For this review, take the finished solid that the model builds, in its own axes (mm). Face numbers are marked on the shaded views. A direction names the side the tool comes from. Give positions to 0.01 mm unless a question says otherwise; leave off trailing zeros. Loops run counter-clockwise (first coordinate to the right, second up) from the corner with the lowest first, then second, coordinate; pieces in that order, holes last. Notation, with made-up numbers: (-11.5, 38.5) - (40.5, 38.5) arc R17 ccw to (40.5, 62.5) - close; hole circle Ø4 at (-11.5, 46.5). An arc over 180 degrees is marked (long way). Answer in a Markdown table with one row per item.
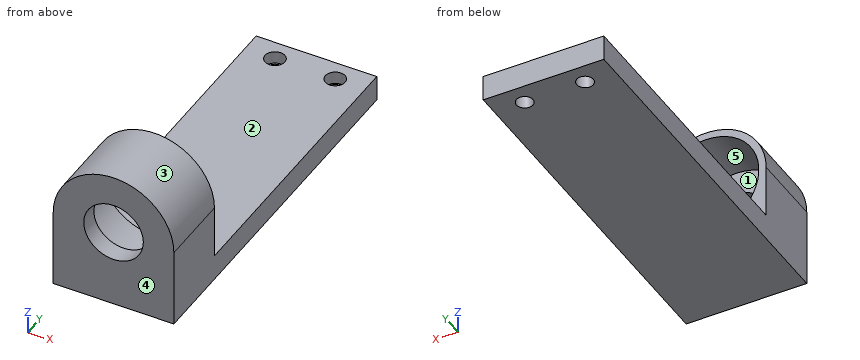
```python
from build123d import *

# Parameters (mm, degrees)
SKETCH1_R                      = 8.1
BOSS_EXTRUDE1_DEPTH            = 100
SKETCH2_R                      = 14.4
CUT_EXTRUDE1_DEPTH             = 80
CUT_EXTRUDE2_START             = -80
CUT_EXTRUDE2_DEPTH             = 80
SKETCH4_R                      = 14.4
CUT_EXTRUDE3_DEPTH             = 15
CBORE_FOR_M4_SHCS1_D           = 4.5
CBORE_FOR_M4_SHCS1_CBORE_D     = 5.4
CBORE_FOR_M4_SHCS1_CBORE_DEPTH = 3.4


with BuildPart() as part:
    # Sketch1 → Boss-Extrude1 (new body)
    with BuildSketch(Plane(origin=(0, 0, 0), x_dir=(1, 0, 0), z_dir=(0, 1, 0))):
        with BuildLine():
            Line((-16.4, 0), (-16.4, 21.4))
            Line((-16.4, 21.4), (16.4, 21.4))
            Line((16.4, 21.4), (16.4, 0))
            ThreePointArc((16.4, 0), (0, -16.4), (-16.4, 0))
        make_face()
        with Locations(Location((0, 0, 0), (0, 0, 270))):
            Circle(SKETCH1_R, mode=Mode.SUBTRACT)
    extrude(amount=BOSS_EXTRUDE1_DEPTH)

    # Sketch2 → Cut-Extrude1 (cut)
    with BuildSketch(Plane(origin=(0, 100, 0), x_dir=(1, 0, 0), z_dir=(0, 1, 0))):
        with Locations(Location((0, 0, 0), (0, 0, 270))):
            Circle(SKETCH2_R)
    extrude(amount=-CUT_EXTRUDE1_DEPTH, mode=Mode.SUBTRACT)

    # Sketch3 → Cut-Extrude2 (cut)
    with BuildSketch(Plane(origin=(0, 100, 0), x_dir=(1, 0, 0), z_dir=(0, 1, 0)).offset(CUT_EXTRUDE2_START)):
        with BuildLine():
            Line((-16.4, 0), (-16.4, 14.4))
            Line((-16.4, 14.4), (16.4, 14.4))
            Line((16.4, 14.4), (16.4, 0))
            ThreePointArc((16.4, 0), (0, -16.4), (-16.4, 0))
        make_face()
    extrude(amount=CUT_EXTRUDE2_DEPTH, mode=Mode.SUBTRACT)

    # Sketch4 → Cut-Extrude3 (cut)
    with BuildSketch(Plane(origin=(0, 20, 0), x_dir=(1, 0, 0), z_dir=(0, 1, 0))):
        with Locations(Location((0, 0, 0), (0, 0, 270))):
            Circle(SKETCH4_R)
    extrude(amount=-CUT_EXTRUDE3_DEPTH, mode=Mode.SUBTRACT)

    # CBORE for M4 SHCS1 (through all)
    with Locations(Plane.XY.offset(-14.4)):
        with Locations((8.2, 94.410911653), (-8.2, 94.410911653)):
            CounterBoreHole(CBORE_FOR_M4_SHCS1_D / 2, CBORE_FOR_M4_SHCS1_CBORE_D / 2, CBORE_FOR_M4_SHCS1_CBORE_DEPTH)


solid = part.part
```
1. We need section D-D, the plane z = -11.5. Give the boundary of the cut face in (x, y), and give its area (3 significant figures).
Values:
| item | result |
|---|---|
| outline | (-16.4, 0) - (16.4, 0) - (16.4, 20) - (8.67, 20) - (8.67, 5) - (-8.67, 5) - (-8.67, 20) - (-16.4, 20) - close |
| area | 396 mm^2 |
2. Wall thickness on line 1 (Z direction, x = 0, y = 11); line 2 (Y direction, x = -8, z = -16); line 3 (Y direction, x = 8.2, z = -19.5): over which ranges is each line inside the solid? List them lowest first. Write a range as [from, to].
Values:
| item | result |
|---|---|
| line 1 | z = [-21.4, -14.4], [14.4, 16.4] |
| line 2 | y = [0, 91.72], [97.1, 100] |
| line 3 | y = [0, 92.16], [96.66, 100] |
3. Clearance check with flat-ended pins moving along their axes: pin 1 (7 mm diameter, centred on x = 8.2, y = 94.41, fed in from +Z); pin 2 (15.5 mm diameter, centred on x = -1, z = -5.5, fed in from +Y); pin 3 (3.5 mm diameter, centred on x = -8.2, y = 94.41, fed in from -Z). State where each tip first meets the part, or that it passes through.
Values:
| item | result |
|---|---|
| pin 1 | stops at z = -14.4 |
| pin 2 | stops at y = 5 |
| pin 3 | passes through |
4. We need section C-C, the plane x = 2. Give the boundary of the cut face in (y, z), and give its area (3 significant figures).
Values:
| item | result |
|---|---|
| outline | (0, -21.4) - (100, -21.4) - (100, -14.4) - (20, -14.4) - (20, -14.26) - (5, -14.26) - (5, -7.85) - (0, -7.85) - close; (0, 7.85) - (5, 7.85) - (5, 14.26) - (20, 14.26) - (20, 16.28) - (0, 16.28) - close |
| area | 807 mm^2 |
5. We need section B-B, the plane x = 7. Give the boundary of the cut face in (y, z).
Values:
| item | result |
|---|---|
| outline | (0, -21.4) - (92.51, -21.4) - (92.51, -17.8) - (91.99, -17.8) - (91.99, -14.4) - (20, -14.4) - (20, -12.58) - (5, -12.58) - (5, -4.08) - (0, -4.08) - close; (0, 4.08) - (5, 4.08) - (5, 12.58) - (20, 12.58) - (20, 14.83) - (0, 14.83) - close; (96.31, -21.4) - (100, -21.4) - (100, -14.4) - (96.83, -14.4) - (96.83, -17.8) - (96.31, -17.8) - close |
6. For the marked faces 4 and 5, list the 3-axis set-ups (+Z, -Z, +X, -X, +Y, -Y) from which the entire face can be reached by the end or side of a thin tool; tool diameter is ignored.
Values:
| item | result |
|---|---|
| face 4 | +Z, -Z, +X, -X, -Y |
| face 5 | +Y |
7. Mouldability with a two-part tool opening along X and no side actions: class the marked faces 1, 2 and 3 as released by +X, released by -X, zero draft, split by the parting line, or undercut.
Values:
| item | result |
|---|---|
| face 1 | undercut |
| face 2 | zero draft |
| face 3 | split by the parting line |
8. We need section A-A, the plane y = 18. Give the boundary of the cut face in (x, z), and give its area (3 significant figures).
Values:
| item | result |
|---|---|
| outline | (-16.4, -21.4) - (16.4, -21.4) - (16.4, 0) arc R16.4 ccw to (-16.4, 0) - close; hole circle Ø28.8 at (0, 0) |
| area | 473 mm^2 |
